Read the model definition and answer for the solid it produces. Units are mm, in the model's axes. A direction names the side the tool comes from. Coordinates: 2 decimals unless noted, no trailing zeros. Order: outer loops, then holes, each group sorted by start corner. A loop starts at its lowest first (then second) coordinate and runs counter-clockwise, first axis right, second up.
from build123d import *

# Parameters (mm, degrees)
F0_W     = 1
F0_H     = 24
F0_H_2   = 1
F0_W_2   = 24
F1_DEPTH = 135
F2_W     = 35
F2_H     = 21.5
F3_DEPTH = 1
F4_W     = 35
F4_H     = 21.5
F4_W_2   = 65
F5_DEPTH = 1


with BuildPart() as f1:
    # F0 (on Right) → F1 (new body)
    with BuildSketch(Plane.YZ):
        with Locations((-64.544081, 31.736633)):
            Rectangle(F0_W, F0_H)
        with Locations((-64.544081, 44.236633)):
            Rectangle(F0_W, F0_H_2)
        with Locations((-52.044081, 44.236633)):
            Rectangle(F0_W_2, F0_H_2)
    extrude(amount=F1_DEPTH)

    # F2 (on face) → F3 (cut)
    with BuildSketch(Plane.XY.offset(44.736633)):
        with Locations((91, -50.794081)):
            Rectangle(F2_W, F2_H)
    extrude(amount=-F3_DEPTH, mode=Mode.SUBTRACT)

    # F4 (on face) → F5 (cut)
    with BuildSketch(Plane.XZ.offset(65.044081)):
        with Locations((91, 30.486633)):
            Rectangle(F4_W, F4_H)
        with Locations((32.5, 30.486633)):
            Rectangle(F4_W_2, F4_H)
    extrude(amount=-F5_DEPTH, mode=Mode.SUBTRACT)


solid = f1.part
Q1. The part is cut by section D-D, the plane x = 117.5. Determine the outline of the cut face in (y, z), then the cut area to 3 significant figures.
Q2. The part is cut by section B-B, the plane z = 39.25. Determine the outline of the cut face in (x, y).
Q3. Which of the six approach directions +Z, -Z, +X, -X, +Y, -Y give full straight-line access (tool end or side, diameter ignored) to faces 1 (the flat face through (0, -54, 44)), 2 (the flat face through (97, -64.044, 42))?
Q4. Straight lines are drawn through the part: L1, parallel to Y at x = 72, z = 23.25; L2, parallel to Z at x = 124.5, y = -41.25. For each, find the intervals that lie inside material, in ascending order.
Q5. The part is cut by section C-C, the plane x = 63.5. Determine the outline of the cut face in (y, z).
Q6. The part is cut by section A-A, the plane y = -42.5. Determine the outline of the cut face in (x, z), then the cut area to 3 significant figures.
Q7. Each of these flat-tipped pins is pushed along its axis until it touches: P1, Ø6, axis at y = -51, z = 40, coming from the +X side; P2, Ø1.5, axis at x = 57, y = -46.5, coming from the -Z side; P3, Ø0.8, axis at y = -64.5, z = 33, coming from the -X side; P4, Ø1.1, axis at x = 95.5, z = 44, coming from the +Y side. Where does it stop, or does it pass through?
Computed values:
1. outline: (-65.04, 19.74) - (-64.04, 19.74) - (-64.04, 43.74) - (-40.04, 43.74) - (-40.04, 44.74) - (-65.04, 44.74) - close
1. area: 49.0 mm2
2. outline: (65, -65.04) - (73.5, -65.04) - (73.5, -64.04) - (65, -64.04) - close; (108.5, -65.04) - (135, -65.04) - (135, -64.04) - (108.5, -64.04) - close
3. face 1: +Z, -Z, -X, +Y, -Y
3. face 2: -Z, +X, -X, +Y
4. L1: y = -65.04 to -64.04
4. L2: z = 43.74 to 44.74
5. outline: (-65.04, 41.24) - (-64.04, 41.24) - (-64.04, 43.74) - (-40.04, 43.74) - (-40.04, 44.74) - (-65.04, 44.74) - close
6. outline: (0, 43.74) - (73.5, 43.74) - (73.5, 44.74) - (0, 44.74) - close; (108.5, 43.74) - (135, 43.74) - (135, 44.74) - (108.5, 44.74) - close
6. area: 100 mm2
7. P1: passes through
7. P2: stops at z = 43.74
7. P3: stops at x = 65
7. P4: stops at y = -61.54
